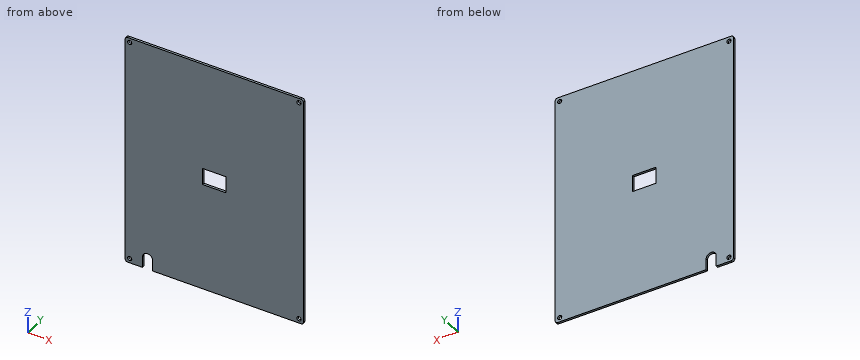
from build123d import *

# Parameters (mm, degrees)
SKETCH1_W           = 160
SKETCH1_H           = 210
BOSS_EXTRUDE1_DEPTH = 2
SKETCH2_R           = 1.9
CUT_EXTRUDE1_DEPTH  = 10
FILLET1_R           = 2
SKETCH3_W           = 21
SKETCH3_H           = 15
CUT_EXTRUDE2_DEPTH  = 10


with BuildPart() as part:
    # Sketch1 → Boss-Extrude1 (new body)
    with BuildSketch(Plane(origin=(0, 0, 0), x_dir=(1, 0, 0), z_dir=(0, 1, 0))):
        with Locations((80, 105)):
            Rectangle(SKETCH1_W, SKETCH1_H)
    extrude(amount=BOSS_EXTRUDE1_DEPTH)

    # Sketch2 → Cut-Extrude1 (cut)
    with BuildSketch(Plane(origin=(0, 2, 0), x_dir=(1, 0, 0), z_dir=(0, 1, 0))):
        with Locations(Location((4, 206, 0), (0, 0, 270))):
            Circle(SKETCH2_R)
        with Locations(Location((156, 206, 0), (0, 0, 90))):
            Circle(SKETCH2_R)
        with Locations(Location((156, 4, 0), (0, 0, 270))):
            Circle(SKETCH2_R)
        with Locations(Location((4, 4, 0), (0, 0, 90))):
            Circle(SKETCH2_R)
        with BuildLine():
            Line((24.5, 200), (24.5, 210))
            Line((24.5, 210), (15.5, 210))
            Line((15.5, 210), (15.5, 200))
            ThreePointArc((15.5, 200), (20, 195.5), (24.5, 200))
        make_face()
    extrude(amount=-CUT_EXTRUDE1_DEPTH, mode=Mode.SUBTRACT)

    # Fillet1
    fillet1_edges = [part.edges().sort_by_distance(p)[0] for p in [
        (0, 1, -210),
        (160, 1, -210),
        (160, 1, 0),
        (0, 1, 0),
    ]]
    fillet(fillet1_edges, radius=FILLET1_R)

    # Sketch3 → Cut-Extrude2 (cut)
    with BuildSketch(Plane(origin=(0, 2, 0), x_dir=(1, 0, 0), z_dir=(0, 1, 0))):
        with Locations((80, 105)):
            Rectangle(SKETCH3_W, SKETCH3_H)
    extrude(amount=-CUT_EXTRUDE2_DEPTH, mode=Mode.SUBTRACT)


solid = part.part
Check sheet for the modelled part. Datum: model origin and axes. Units: mm. Round coordinates to 2 decimals unless told otherwise and drop trailing zeros. Loops run counter-clockwise (first coordinate to the right, second up) from the corner with the lowest first, then second, coordinate; pieces in that order, holes last.
1. Scan lines: probe 1 along X at (y, z) = (1.2, -4); probe 2 along Z at (x, y) = (156, 1.65); probe 3 along X at (y, z) = (1.2, -111.5). Record each from-to range of solid material in increasing order.
2. Sectioned sample at A-A on x = 85. Record the boundary of the cut face in (y, z), and give its area (3 significant figures).
3. Sectioned sample at B-B on x = 20. Record the boundary of the cut face in (y, z), and give its area (3 significant figures).
Recorded:
1. probe 1: x = 0 to 2.1, 5.9 to 154.1, 157.9 to 160
1. probe 2: z = -210 to -207.9, -204.1 to -5.9, -2.1 to 0
1. probe 3: x = 0 to 69.5, 90.5 to 160
2. outline: (0, -210) - (2, -210) - (2, -112.5) - (0, -112.5) - close; (0, -97.5) - (2, -97.5) - (2, 0) - (0, 0) - close
2. area: 390 mm2
3. outline: (0, -195.5) - (2, -195.5) - (2, 0) - (0, 0) - close
3. area: 391 mm2
